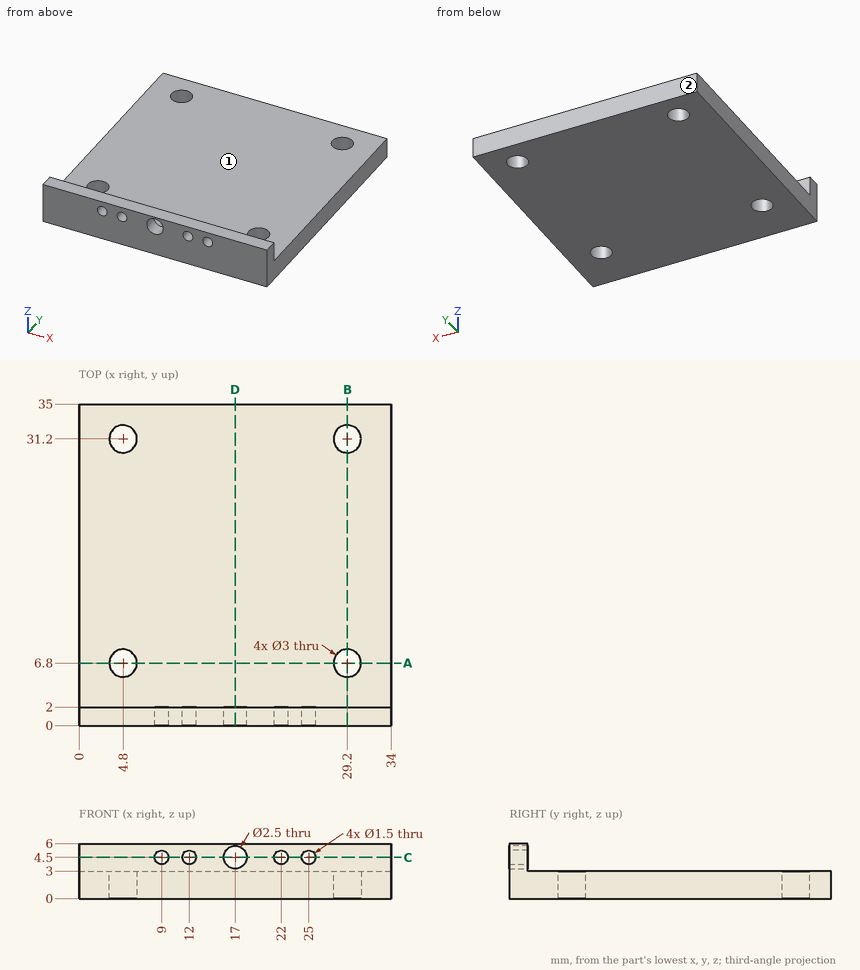
For this review, use the dimensioned drawing (mm, ordinates from the lowest corner) and the shaded views. A direction names the side the tool comes from. Round coordinates to 2 decimals unless told otherwise and drop trailing zeros. Write each loop counter-clockwise with the first axis right and the second up, starting at its lowest first coordinate (ties: lowest second). Pieces come first, ordered by that corner, then holes. Notation, with made-up numbers: (78, 1) - (124, 1) arc R8 cw to (124, 13) - close; hole circle Ø5 at (32.25, 46.25). An arc over 180 degrees is marked (long way). One line per item, written item: value. Start each with the question number.
1. Consider section D-D on x = 17. Write out the cut boundary in (y, z).
2. To check wall thickness, follow L1, parallel to X at y = 0.65, z = 4.5; L2, parallel to Y at x = 29.2, z = 0.75; L3, parallel to Y at x = 30, z = 0.55. State the ranges of each line that lie inside material, in increasing order. Write a range as from..to.
3. Consider section C-C on z = 4.5. Write out the cut boundary in (x, y).
4. Machinability: for the marked faces 1 and 2, which of the approach directions +Z, -Z, +X, -X, +Y, -Y give a long, thin tool a straight path to every point of the face, cutting with its end or side? Answer none if there is none.
5. Consider section A-A on y = 6.8. Write out the cut boundary in (x, z), and give its area (3 significant figures).
6. Clearance check with flat-ended pins moving along their axes: P1, Ø2.5, axis at x = 19.5, z = 5, coming from the +Y side; P2, Ø1.5, axis at x = 9, y = 7, coming from the +Z side. State where each tip first meets the part, or that it passes through.
7. Consider section B-B on x = 29.2. Write out the cut boundary in (y, z), and give its area (3 significant figures).
Checks:
1. outline: (0, 0) - (35, 0) - (35, 3) - (2, 3) - (2, 3.25) - (0, 3.25) - close; (0, 5.75) - (2, 5.75) - (2, 6) - (0, 6) - close
2. L1: x = 0..8.25, 9.75..11.25, 12.75..15.75, 18.25..21.25, 22.75..24.25, 25.75..34
2. L2: y = 0..5.3, 8.3..29.7, 32.7..35
2. L3: y = 0..5.53, 8.07..29.93, 32.47..35
3. outline: (0, 0) - (8.25, 0) - (8.25, 2) - (0, 2) - close; (9.75, 0) - (11.25, 0) - (11.25, 2) - (9.75, 2) - close; (12.75, 0) - (15.75, 0) - (15.75, 2) - (12.75, 2) - close; (18.25, 0) - (21.25, 0) - (21.25, 2) - (18.25, 2) - close; (22.75, 0) - (24.25, 0) - (24.25, 2) - (22.75, 2) - close; (25.75, 0) - (34, 0) - (34, 2) - (25.75, 2) - close
4. face 1: +Z, +X, -X, +Y
4. face 2: +Z, -Z, +X, -X, +Y
5. outline: (0, 0) - (3.3, 0) - (3.3, 3) - (0, 3) - close; (6.3, 0) - (27.7, 0) - (27.7, 3) - (6.3, 3) - close; (30.7, 0) - (34, 0) - (34, 3) - (30.7, 3) - close
5. area: 84.0 mm^2
6. P1: stops at y = 2
6. P2: stops at z = 3
7. outline: (0, 0) - (5.3, 0) - (5.3, 3) - (2, 3) - (2, 6) - (0, 6) - close; (8.3, 0) - (29.7, 0) - (29.7, 3) - (8.3, 3) - close; (32.7, 0) - (35, 0) - (35, 3) - (32.7, 3) - close
7. area: 93.0 mm^2
